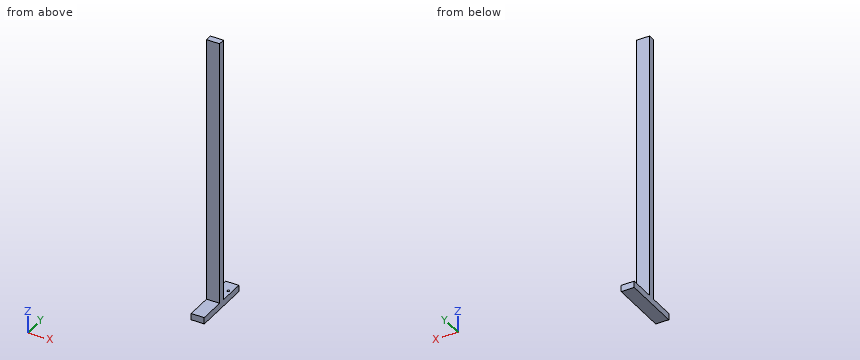
```python
from build123d import *

# Parameters (mm, degrees)
F0_W          = 76.2
F0_H          = 38.1
F1_DEPTH      = 1568.45
F2_W          = 76.2
F2_H          = 38.1
F3_DEPTH      = 38.1
F4_W          = 76.2
F4_H          = 38.1
F5_DEPTH      = 152.4
F5_DEPTH_BACK = 190.5
F6_R          = 6.35
F7_DEPTH      = 2.54


with BuildPart() as f1:
    # F0 (on Top) → F1 (new body)
    with BuildSketch(Plane.XY):
        Rectangle(F0_W, F0_H)
    extrude(amount=F1_DEPTH)

    # F2 (on face) → F3 (join)
    with BuildSketch(Plane(origin=(0, 0, 0), x_dir=(1, 0, 0), z_dir=(0, 0, -1))):
        Rectangle(F2_W, F2_H)
    extrude(amount=F3_DEPTH)

    # F4 (on face) → F5 (join, two sides)
    with BuildSketch(Plane.XZ.offset(19.05)) as f5_sk:
        with Locations((0, -19.05)):
            Rectangle(F4_W, F4_H)
    extrude(amount=F5_DEPTH)
    extrude(f5_sk.sketch, amount=-F5_DEPTH_BACK)

    # F6 (on face) → F7 (join)
    with BuildSketch(Plane.XY):
        with Locations((19.05, 99.86645)):
            Circle(F6_R)
    extrude(amount=F7_DEPTH)


solid = f1.part
```
Check sheet for the modelled part. Datum: model origin and axes. Units: mm. Give positions to 0.01 mm unless a question says otherwise; leave off trailing zeros. Order: outer loops, then holes, each group sorted by start corner. A loop starts at its lowest first (then second) coordinate and runs counter-clockwise, first axis right, second up. Notation, with made-up numbers: (82, 54) -> (108, 54) arc R28 cw to (108, 79) -> close; hole circle Ø9 at (64.5, 56). An arc over 180 degrees is marked (long way). Use CSV: the item, a comma, the result in double quotes. Start each with the question number.
1) Sectioned sample at A-A, the plane x = -14. Record the boundary of the cut face in (y, z), plus the area to 3 significant figures.
2) Sectioned sample at C-C, the plane y = 42. Record the boundary of the cut face in (x, z), plus the area to 3 significant figures.
3) Sectioned sample at B-B, the plane z = 901. Record the boundary of the cut face in (x, y).
4) Go/stop test with flat-tipped pins: P1, Ø14, axis at x = 19.5, y = 98.5, coming from the +Z side; P2, Ø4, axis at x = -4, z = 751, coming from the +Y side; P3, Ø8, axis at x = 25, y = -82.5, coming from the +Z side. Record where each tip stops, or that it passes through.
5) Material ranges on line 1 (Z direction, x = -35, y = -54.5); line 2 (Y direction, x = -28, z = 1225), recorded low to high. Write a range as from..to.
Recorded:
1,outline,"(-171.45, -38.1) -> (171.45, -38.1) -> (171.45, 0) -> (19.05, 0) -> (19.05, 1568.45) -> (-19.05, 1568.45) -> (-19.05, 0) -> (-171.45, 0) -> close"
1,area,"72,800 mm2"
2,outline,"(-38.1, -38.1) -> (38.1, -38.1) -> (38.1, 0) -> (-38.1, 0) -> close"
2,area,"2,900 mm2"
3,outline,"(-38.1, -19.05) -> (38.1, -19.05) -> (38.1, 19.05) -> (-38.1, 19.05) -> close"
4,P1,"z = 2.54"
4,P2,"y = 19.05"
4,P3,"z = 0"
5,line 1,"-38.1..0"
5,line 2,"-19.05..19.05"
